from build123d import *

# Parameters (mm, degrees)
SKETCH1_R           = 9
SKETCH1_R_2         = 1.2
BOSS_EXTRUDE1_DEPTH = 5
SKETCH2_R           = 24
BOSS_EXTRUDE2_DEPTH = 1.2
SKETCH4_R           = 1.2
CUT_EXTRUDE1_DEPTH  = 35.307433597
SKETCH5_R           = 10
SKETCH5_R_2         = 1.2
BOSS_EXTRUDE4_DEPTH = 2
SKETCH6_R           = 24
SKETCH6_R_2         = 22.8
BOSS_EXTRUDE5_DEPTH = 10
SKETCH7_W           = 12
SKETCH7_H           = 48
CUT_EXTRUDE2_DEPTH  = 2
BOSS_EXTRUDE6_START = -3
SKETCH9_R           = 1.6
BOSS_EXTRUDE6_DEPTH = 3
SKETCH10_R          = 2.5
CUT_EXTRUDE3_DEPTH  = 7
BOSS_EXTRUDE7_START = -1
SKETCH1_2_R         = 9
SKETCH1_2_R_2       = 1.2
BOSS_EXTRUDE7_DEPTH = 1
CUT_EXTRUDE4_DEPTH  = 5
SKETCH18_OUTSIDE_W  = 64.006
SKETCH18_OUTSIDE_H  = 64.006
SKETCH18_OUTSIDE_R  = 24
CUT_EXTRUDE5_DEPTH  = 5


with BuildPart() as part:
    # Sketch1 → Boss-Extrude1 (new body)
    with BuildSketch(Plane(origin=(0, 0, 0), x_dir=(1, 0, 0), z_dir=(0, 1, 0))):
        with Locations(Location((0, 0, 0), (0, 0, 270))):
            Circle(SKETCH1_R)
        with Locations(Location((4.242640687, 4.242640687, 0), (0, 0, 270))):
            Circle(SKETCH1_R_2, mode=Mode.SUBTRACT)
        with Locations(Location((-4.242640687, 4.242640687, 0), (0, 0, 270))):
            Circle(SKETCH1_R_2, mode=Mode.SUBTRACT)
        with Locations(Location((4.242640687, -4.242640687, 0), (0, 0, 270))):
            Circle(SKETCH1_R_2, mode=Mode.SUBTRACT)
        with Locations(Location((-4.242640687, -4.242640687, 0), (0, 0, 270))):
            Circle(SKETCH1_R_2, mode=Mode.SUBTRACT)
    extrude(amount=BOSS_EXTRUDE1_DEPTH)

    # Sketch2 → Boss-Extrude2 (add)
    with BuildSketch(Plane(origin=(0, 5, 0), x_dir=(1, 0, 0), z_dir=(0, 1, 0))):
        with Locations(Location((0, 0, 0), (0, 0, 270))):
            Circle(SKETCH2_R)
    extrude(amount=BOSS_EXTRUDE2_DEPTH)

    # Sketch4 → Cut-Extrude1 (cut, through all)
    with BuildSketch(Plane.XZ.offset(-5)):
        with Locations(Location((-4.242640687, -4.242640687, 0), (0, 0, 270))):
            Circle(SKETCH4_R)
        with Locations(Location((4.242640687, -4.242640687, 0), (0, 0, 270))):
            Circle(SKETCH4_R)
        with Locations(Location((4.242640687, 4.242640687, 0), (0, 0, 270))):
            Circle(SKETCH4_R)
        with Locations(Location((-4.242640687, 4.242640687, 0), (0, 0, 270))):
            Circle(SKETCH4_R)
    extrude(amount=-CUT_EXTRUDE1_DEPTH, mode=Mode.SUBTRACT)

    # Sketch5 → Boss-Extrude4 (add)
    with BuildSketch(Plane(origin=(0, 6.2, 0), x_dir=(1, 0, 0), z_dir=(0, 1, 0))):
        with Locations(Location((0, 0, 0), (0, 0, 270))):
            Circle(SKETCH5_R)
        with Locations(Location((4.242640687, -4.242640687, 0), (0, 0, 270))):
            Circle(SKETCH5_R_2, mode=Mode.SUBTRACT)
        with Locations(Location((-4.242640687, -4.242640687, 0), (0, 0, 270))):
            Circle(SKETCH5_R_2, mode=Mode.SUBTRACT)
        with Locations(Location((-4.242640687, 4.242640687, 0), (0, 0, 270))):
            Circle(SKETCH5_R_2, mode=Mode.SUBTRACT)
        with Locations(Location((4.242640687, 4.242640687, 0), (0, 0, 270))):
            Circle(SKETCH5_R_2, mode=Mode.SUBTRACT)
    extrude(amount=BOSS_EXTRUDE4_DEPTH)

    # Sketch6 → Boss-Extrude5 (add)
    with BuildSketch(Plane(origin=(0, 6.2, 0), x_dir=(1, 0, 0), z_dir=(0, 1, 0))):
        with Locations(Location((0, 0, 0), (0, 0, 270))):
            Circle(SKETCH6_R)
        with Locations(Location((0, 0, 0), (0, 0, 270))):
            Circle(SKETCH6_R_2, mode=Mode.SUBTRACT)
    extrude(amount=BOSS_EXTRUDE5_DEPTH)

    # Sketch7 → Cut-Extrude2 (cut)
    with BuildSketch(Plane(origin=(0, 16.2, 0), x_dir=(1, 0, 0), z_dir=(0, 1, 0))):
        Rectangle(SKETCH7_W, SKETCH7_H)
    extrude(amount=-CUT_EXTRUDE2_DEPTH, mode=Mode.SUBTRACT)

    # Sketch9 → Boss-Extrude6 (add)
    # profile 1 of 4: a face of its own
    with BuildSketch(Plane(origin=(0, 16.2, 0), x_dir=(1, 0, 0), z_dir=(0, 1, 0)).offset(BOSS_EXTRUDE6_START)):
        with BuildLine():
            Line((-11, -14.996363336), (-11, -19.970978944))
            ThreePointArc((-11, -19.970978944), (-8.560113637, -21.132071704), (-6, -21.996363336))
            Line((-6, -21.996363336), (-6, -14.996363336))
            Line((-6, -14.996363336), (-11, -14.996363336))
        make_face()
        with Locations(Location((-8.5, -17.5, 0), (0, 0, 270))):
            Circle(SKETCH9_R, mode=Mode.SUBTRACT)
    # profile 2 of 4: a face of its own
    with BuildSketch(Plane(origin=(0, 16.2, 0), x_dir=(1, 0, 0), z_dir=(0, 1, 0)).offset(BOSS_EXTRUDE6_START)):
        with BuildLine():
            ThreePointArc((6, -21.996363336), (8.560113637, -21.132071704), (11, -19.970978944))
            Line((11, -19.970978944), (11, -14.996363336))
            Line((11, -14.996363336), (6, -14.996363336))
            Line((6, -14.996363336), (6, -21.996363336))
        make_face()
        with Locations(Location((8.5, -17.5, 0), (0, 0, 270))):
            Circle(SKETCH9_R, mode=Mode.SUBTRACT)
    # profile 3 of 4: a face of its own
    with BuildSketch(Plane(origin=(0, 16.2, 0), x_dir=(1, 0, 0), z_dir=(0, 1, 0)).offset(BOSS_EXTRUDE6_START)):
        with BuildLine():
            ThreePointArc((11, 19.970978944), (8.560113637, 21.132071704), (6, 21.996363336))
            Line((6, 21.996363336), (6, 14.996363336))
            Line((6, 14.996363336), (11, 14.996363336))
            Line((11, 14.996363336), (11, 19.970978944))
        make_face()
        with Locations(Location((8.5, 17.5, 0), (0, 0, 270))):
            Circle(SKETCH9_R, mode=Mode.SUBTRACT)
    # profile 4 of 4: a face of its own
    with BuildSketch(Plane(origin=(0, 16.2, 0), x_dir=(1, 0, 0), z_dir=(0, 1, 0)).offset(BOSS_EXTRUDE6_START)):
        with BuildLine():
            Line((-6, 14.996363336), (-6, 21.996363336))
            ThreePointArc((-6, 21.996363336), (-8.560113637, 21.132071704), (-11, 19.970978944))
            Line((-11, 19.970978944), (-11, 14.996363336))
            Line((-11, 14.996363336), (-6, 14.996363336))
        make_face()
        with Locations(Location((-8.5, 17.5, 0), (0, 0, 270))):
            Circle(SKETCH9_R, mode=Mode.SUBTRACT)
    extrude(amount=BOSS_EXTRUDE6_DEPTH)

    # Sketch10 → Cut-Extrude3 (cut)
    with BuildSketch(Plane(origin=(0, 8.2, 0), x_dir=(1, 0, 0), z_dir=(0, 1, 0))):
        with Locations(Location((4.242640687, 4.242640687, 0), (0, 0, 270))):
            Circle(SKETCH10_R)
        with Locations(Location((4.242640687, -4.242640687, 0), (0, 0, 270))):
            Circle(SKETCH10_R)
        with Locations(Location((-4.242640687, -4.242640687, 0), (0, 0, 270))):
            Circle(SKETCH10_R)
        with Locations(Location((-4.242640687, 4.242640687, 0), (0, 0, 270))):
            Circle(SKETCH10_R)
    extrude(amount=-CUT_EXTRUDE3_DEPTH, mode=Mode.SUBTRACT)

    # Sketch1_2 → Boss-Extrude7 (add)
    with BuildSketch(Plane(origin=(0, 0, 0), x_dir=(1, 0, 0), z_dir=(0, 1, 0)).offset(BOSS_EXTRUDE7_START)):
        with Locations(Location((0, 0, 0), (0, 0, 270))):
            Circle(SKETCH1_2_R)
        with Locations(Location((4.242640687, 4.242640687, 0), (0, 0, 270))):
            Circle(SKETCH1_2_R_2, mode=Mode.SUBTRACT)
        with Locations(Location((-4.242640687, 4.242640687, 0), (0, 0, 270))):
            Circle(SKETCH1_2_R_2, mode=Mode.SUBTRACT)
        with Locations(Location((4.242640687, -4.242640687, 0), (0, 0, 270))):
            Circle(SKETCH1_2_R_2, mode=Mode.SUBTRACT)
        with Locations(Location((-4.242640687, -4.242640687, 0), (0, 0, 270))):
            Circle(SKETCH1_2_R_2, mode=Mode.SUBTRACT)
    extrude(amount=BOSS_EXTRUDE7_DEPTH)

    # Sketch15 → Cut-Extrude4 (cut)
    with BuildSketch(Plane(origin=(18.32105018, 1.602e-06, -18.32105018), x_dir=(-0.7071067811865515, 6.181721199999928e-08, -0.7071067811865409), z_dir=(0.7071067811865437, 6.181721199999997e-08, -0.7071067811865488))):
        with BuildLine():
            Line((-4.091985108, 11.979999846), (2.848014892, 11.979998988))
            ThreePointArc((2.848014892, 11.979998988), (4.241015323, 12.556998456), (4.818015136, 13.949998744))
            Line((4.818015136, 13.949998744), (4.818015284, 15.149998744))
            ThreePointArc((4.818015284, 15.149998744), (4.241015815, 16.542999174), (2.848015528, 17.119998988))
            Line((2.848015528, 17.119998988), (-4.091984472, 17.119999846))
            ThreePointArc((-4.091984472, 17.119999846), (-5.484984903, 16.543000377), (-6.061984716, 15.150000089))
            Line((-6.061984716, 15.150000089), (-6.061984864, 13.950000089))
            ThreePointArc((-6.061984864, 13.950000089), (-5.484985395, 12.556999659), (-4.091985108, 11.979999846))
        make_face()
    extrude(amount=-CUT_EXTRUDE4_DEPTH, mode=Mode.SUBTRACT)

    # Sketch18 outside → Cut-Extrude5 (cut)
    # profile 1 of 2: a face of its own
    with BuildSketch(Plane(origin=(0, 16.2, 0), x_dir=(1, 0, 0), z_dir=(0, 1, 0))):
        Rectangle(SKETCH18_OUTSIDE_W, SKETCH18_OUTSIDE_H)
        with Locations(Location((0, 0, 0), (0, 0, 104.477512186))):
            Circle(SKETCH18_OUTSIDE_R, mode=Mode.SUBTRACT)
    # profile 2 of 2: a face of its own
    with BuildSketch(Plane(origin=(0, 16.2, 0), x_dir=(1, 0, 0), z_dir=(0, 1, 0))):
        Polygon((11, 16.996363336), (9, 14.996363336), (11, 14.996363336), align=None)
    extrude(amount=-CUT_EXTRUDE5_DEPTH, mode=Mode.SUBTRACT)


solid = part.part
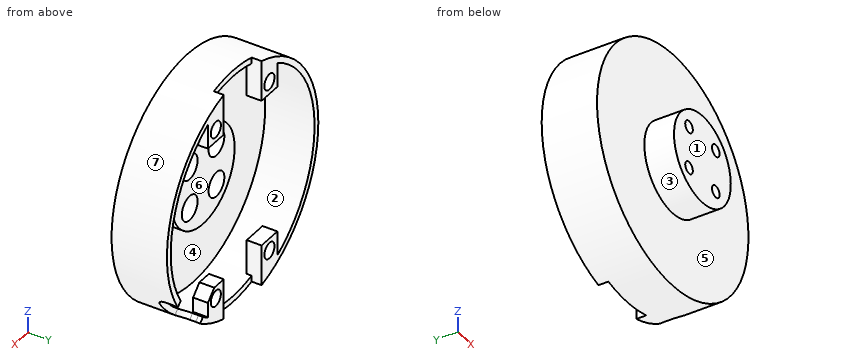
Verification items for the finished model (mm, model axes). Face numbers are marked on the shaded views. A direction names the side the tool comes from. Give positions to 0.01 mm unless a question says otherwise; leave off trailing zeros. Write each loop counter-clockwise with the first axis right and the second up, starting at its lowest first coordinate (ties: lowest second). Pieces come first, ordered by that corner, then holes. Notation, with made-up numbers: M 42,47.25 L 80,47.25 A22 ccw 80,82.25 Z; hole C 83.5,-8 d11. An arc over 180 degrees is marked long. Write item = value, one per line.
(1) Sectioned sample at A-A (z = 17.5). Record the cut outline in (x, y), then the cut area to 3 significant figures.
Found:
outline = M -16.42,5 L 16.42,5 L 16.42,16.2 L 14.61,16.2 L 14.61,6.2 L -14.61,6.2 L -14.61,16.2 L -16.42,16.2 Z; M -11,13.2 L -10.1,13.2 L -10.1,16.2 L -11,16.2 Z; M -6.9,13.2 L -6,13.2 L -6,16.2 L -6.9,16.2 Z; M 6,13.2 L 6.9,13.2 L 6.9,16.2 L 6,16.2 Z; M 10.1,13.2 L 11,13.2 L 11,16.2 L 10.1,16.2 Z
area = 86.4 mm2
(2) Draft check along X on the marked faces 1, 2, 3 and 4. Enter one of: released by +X, released by -X, zero draft, split by the parting line, or undercut.
Found:
face_1 = zero draft
face_2 = undercut
face_3 = split by the parting line
face_4 = undercut
(3) Go/stop test with flat-tipped pins: pin 1 Ø1.5 at (x, z) = (11.5, -13.5) entering from -Y; pin 2 Ø4 at (x, z) = (4.24, -4.24) entering from +Y; pin 3 Ø1 at (y, z) = (1, -3.5) entering from +X. Record where each tip stops, or that it passes through.
Found:
pin_1 = 5
pin_2 = 1.2
pin_3 = 8.49
(4) Sectioned sample at D-D (y = 2.5). Record the cut outline in (x, z), then the cut area to 3 significant figures.
Found:
outline = C 0,0 d18; hole C -4.24,-4.24 d5; hole C -4.24,4.24 d5; hole C 4.24,-4.24 d5; hole C 4.24,4.24 d5
area = 176 mm2
(5) Sectioned sample at C-C (z = 0). Record the cut outline in (x, y), then the cut area to 3 significant figures.
Found:
outline = M -24,5 L -9,5 L -9,-1 L 9,-1 L 9,5 L 24,5 L 24,16.2 L 22.8,16.2 L 22.8,6.2 L 10,6.2 L 10,8.2 L -10,8.2 L -10,6.2 L -22.8,6.2 L -22.8,16.2 L -24,16.2 Z
area = 230 mm2
(6) Sectioned sample at B-B (x = 0). Record the cut outline in (y, z), then the cut area to 3 significant figures.
Found:
outline = M -1,-9 L 5,-9 L 5,-24 L 14.2,-24 L 14.2,-22.8 L 6.2,-22.8 L 6.2,-10 L 8.2,-10 L 8.2,10 L 6.2,10 L 6.2,22.8 L 14.2,22.8 L 14.2,24 L 5,24 L 5,9 L -1,9 Z
area = 225 mm2
(7) Access from +Z, -Z, +X, -X, +Y, -Y to the whole of each face (thin tool, end or side, straight path). Record for the marked faces 5, 6 and 7.
Found:
face_5 = -Y
face_6 = +Y
face_7 = +Y, -Y
(8) Material ranges on line 1 (X direction, y = 14.5, z = 0.5); line 2 (X direction, y = 15.2, z = -17.5); line 3 (Z direction, x = -4, y = 4), recorded low to high.
Found:
line_1 = -23.99 to -22.79, 22.79 to 23.99
line_2 = -16.42 to -14.61, -11 to -10.1, -6.9 to -6, 6 to 6.9, 10.1 to 11
line_3 = -8.06 to -6.73, -1.75 to 1.75, 6.73 to 8.06
